Build history of the part. All positions in model axes, mm. Coordinates: 2 decimals unless noted, no trailing zeros. Loops run counter-clockwise (first coordinate to the right, second up) from the corner with the lowest first, then second, coordinate; pieces in that order, holes last.
(1) Two-plate mould, pull along Z, no slides. Class faces 1 (the face through (2.703, 3.944, 8.584)), 2 (the face through (0, 4, -22.5)), 3 (the face through (18.45, 3.94, 18.1)), 4 (the face through (21, 4.06, 21.07)): pulls with the +Z half, pulls with the -Z half, needs draft (parallel to the pull), parting line crosses it, or undercut.
(2) Wall check: L1, parallel to X at y = 6, z = -17.5 (3 decimals); L2, parallel to X at y = 3, z = 0; L3, parallel to Z at x = 18.5, y = 6.5. Give the ranges that are in metal, low to high.
(3) Slice it at C-C (y = 3.25). Give the cut face in (x, z) (3 decimals), and give its area (3 significant figures).
(4) Slice it at A-A (z = 0). Give the cut face in (x, y).
(5) Slice it at B-B (x = -7). Give the cut face in (y, z).
(6) Flat gauge pins, fed straight in: P1, Ø1.8, axis at x = 17.5, z = -17.5, coming from the +Y side; P2, Ø5, axis at x = 16.5, z = 9.5, coming from the -Y side. Where does each tip first touch, or does it go through?
from build123d import *

# Parameters (mm, degrees)
SKETCH1_W           = 45
SKETCH1_H           = 45
SKETCH1_R           = 9
SKETCH1_R_2         = 1.125
BOSS_EXTRUDE1_DEPTH = 8
FILLET1_R           = 5


with BuildPart() as part:
    # Sketch1 → Boss-Extrude1 (new body)
    with BuildSketch(Plane(origin=(0, 0, 0), x_dir=(1, 0, 0), z_dir=(0, 1, 0))):
        Rectangle(SKETCH1_W, SKETCH1_H)
        with Locations(Location((0, 0, 0), (0, 0, 270))):
            Circle(SKETCH1_R, mode=Mode.SUBTRACT)
        with Locations(Location((-17.5, 17.5, 0), (0, 0, 270))):
            Circle(SKETCH1_R_2, mode=Mode.SUBTRACT)
        with Locations(Location((17.5, 17.5, 0), (0, 0, 270))):
            Circle(SKETCH1_R_2, mode=Mode.SUBTRACT)
        with Locations(Location((17.5, -17.5, 0), (0, 0, 270))):
            Circle(SKETCH1_R_2, mode=Mode.SUBTRACT)
        with Locations(Location((-17.5, -17.5, 0), (0, 0, 270))):
            Circle(SKETCH1_R_2, mode=Mode.SUBTRACT)
    extrude(amount=BOSS_EXTRUDE1_DEPTH)

    # Fillet1
    fillet1_edges = [part.edges().sort_by_distance(p)[0] for p in [
        (-22.5, 4, 22.5),
        (-22.5, 4, -22.5),
        (22.5, 4, -22.5),
        (22.5, 4, 22.5),
    ]]
    fillet(fillet1_edges, radius=FILLET1_R)


solid = part.part
Response values:
1. face 1: undercut
1. face 2: pulls with the -Z half
1. face 3: undercut
1. face 4: pulls with the +Z half
2. L1: x = -22.5 to -18.625, -16.375 to 16.375, 18.625 to 22.5
2. L2: x = -22.5 to -9, 9 to 22.5
2. L3: z = -22.4 to -18.02, -16.98 to 16.98, 18.02 to 22.4
3. outline: (-22.5, -17.5) arc R5 ccw to (-17.5, -22.5) - (17.5, -22.5) arc R5 ccw to (22.5, -17.5) - (22.5, 17.5) arc R5 ccw to (17.5, 22.5) - (-17.5, 22.5) arc R5 ccw to (-22.5, 17.5) - close; hole circle Ø2.25 at (-17.5, -17.5); hole circle Ø2.25 at (-17.5, 17.5); hole circle Ø18 at (0, 0); hole circle Ø2.25 at (17.5, -17.5); hole circle Ø2.25 at (17.5, 17.5)
3. area: 1,730 mm2
4. outline: (-22.5, 0) - (-9, 0) - (-9, 8) - (-22.5, 8) - close; (9, 0) - (22.5, 0) - (22.5, 8) - (9, 8) - close
5. outline: (0, -22.5) - (8, -22.5) - (8, -5.66) - (0, -5.66) - close; (0, 5.66) - (8, 5.66) - (8, 22.5) - (0, 22.5) - close
6. P1: passes through
6. P2: stops at y = 0
